Autodesk Inventor part; units mm, degrees
ref_plane "YZ Plane" through (0, 0, 0) normal (1, 0, 0) x (0, 1, 0)
ref_plane "XZ Plane" through (0, 0, 0) normal (0, 1, 0) x (-1, 0, 0)
ref_plane "XY Plane" through (0, 0, 0) normal (0, 0, 1) x (1, 0, 0)
sketch "Szkic1" plane through (0, 0, 0) normal (0, 0, 1) x (1, 0, 0)
  circle A0 centre (0, 0) radius 10
  dimension "d0" = 20
extrude "Wyciągnięcie proste1" add sketch "Szkic1" along normal blind 430
shell "Skorupa1" thickness 2 removed faces 2 at (-1.182, 3.1167, 430) at (-1.182, 3.1167, 0)
sketch "Szkic2" plane through (0, 0, 0) normal (1, 0, 0) x (0, 1, 0)
  line L0 (-34.5081, 100) -> (42.8278, 100)
  line L1 (-10, 0) -> (10, 0)
  line L2 (10, 430) -> (-10, 430)
  point P0 (0, 0)
  dimension "d4" = 100
bend part "Gięcie części1" radius 25.4648 angle 45 line through (0, -34.5081, 100) along (0, 1, 0) centre toward (1, 0, 0) moving side (0, 0, -1) both sides no
sketch "Szkic3" plane through (0, 0, 0) normal (1, 0, 0) x (0, 1, 0)
  line L0 (-35.2697, 330) -> (39.6293, 330)
  line L1 (10, 430) -> (-10, 430)
  point P0 (0, 0)
  dimension "d8" = 100
bend part "Gięcie części2" radius 25.4648 angle 45 line through (0, -35.2697, 330) along (0, 1, 0) centre toward (1, 0, 0) moving side (0, 0, 1) both sides no
sketch "Szkic4" plane through (0, 0, 0) normal (0, 1, 0) x (-1, 0, 0)
  line L0 (-71.0981, 32.4962) -> (-56.9559, 18.3541) construction
  line L1 (-56.9559, 18.3541) -> (-0.3874, 74.9226) construction
  line L2 (-56.9559, 18.3541) -> (-56.9559, 46.6383)
  line L3 (-71.0981, 32.4962) -> (-14.5295, 89.0647) construction
  line L4 (-56.9559, 46.6383) -> (-71.0981, 32.4962)
  line L5 (-71.0981, 32.4962) -> (-56.9559, 18.3541)
  line L6 (-56.9559, 411.6459) -> (-71.0981, 397.5038) construction
  line L7 (-14.5295, 340.9353) -> (-71.0981, 397.5038) construction
  line L8 (-0.3874, 355.0774) -> (-56.9559, 411.6459) construction
  line L9 (-56.9559, 411.6459) -> (-56.9559, 383.3617)
  line L10 (-56.9559, 383.3617) -> (-71.0981, 397.5038)
  line L11 (-71.0981, 397.5038) -> (-56.9559, 411.6459)
  point P0 (0, 0)
extrude "Wyciągnięcie proste3" cut sketch "Szkic4" along normal mid plane 32
equation "\"PromieńGięcia\" = Grubość"
equation "\"SzerokośćGięciaPodcięcia\" = Grubość"
equation "\"GłębokośćGięciaPodcięcia\" = 0.5 * Grubość"
equation "\"RozmiarPodcięciaNarożnika\" = 4 * Grubość"
equation "\"MinimalnaPozostałość\" = 2 * Grubość"
equation "\"PromieńPrzejścia\" = PromieńGięcia"
equation "\"Rozmiar_promienia_Jacobiego\" = Grubość"
equation "\"Wielk_odstępu\" = Grubość"
properties part number "Rura_poprzeczna_wygieta" material "Aluminium AW-7020"
Can you work these out from the model? Positions are in its coordinate system, mm. A direction names the side the tool comes from. Give positions to 0.01 mm unless a question says otherwise; leave off trailing zeros. Order: outer loops, then holes, each group sorted by start corner. A loop starts at its lowest first (then second) coordinate and runs counter-clockwise, first axis right, second up. Notation, with made-up numbers: M 25,86 L 36,86 A16 ccw 36,109 Z; hole C 88.5,-13 d4. An arc over 180 degrees is marked long. One line per question, with ' | ' between items.
Item 1: We'd pull the mould along X, two halves only. Please class faces 3 (the face through (-1.73, 7.81, 213.39)), 4 (the face through (56.956, -8.2, 32.4)), 5 (the face through (29.81, -0.35, 48.34)), 6 (the face through (22.789, -0.44, 52.534)): released by +X, released by -X, zero draft, split by the parting line, or undercut.
Answer block:
face 3: undercut | face 4: released by +X | face 5: undercut | face 6: split by the parting line
Item 2: Suppose I cut it at B-B, the plane y = 4.75. Write out the boundary of the cut face in (x, z).
Answer block:
outline: M -8.8,100 A34.26 ccw 1.24,75.77 L 56.96,20.05 L 56.96,23.39 L 2.91,77.44 A31.9 cw -6.44,100 L -6.44,330 A31.9 cw 2.91,352.56 L 56.96,406.61 L 56.96,409.95 L 1.24,354.23 A34.26 ccw -8.8,330 Z; M 6.44,100 A19.03 ccw 12.01,86.55 L 56.96,41.6 L 56.96,44.94 L 13.68,88.22 A16.66 cw 8.8,100 L 8.8,330 A16.66 cw 13.68,341.78 L 56.96,385.06 L 56.96,388.4 L 12.01,343.45 A19.03 ccw 6.44,330 Z
Item 3: Suppose I cut it at A-A, the plane z = 207. Write out the boundary of the cut face in (x, y).
Answer block:
outline: C 0,0 d20; hole C 0,0 d16
Item 4: Suppose I cut it at C-C, the plane x = 39.5. Give the number of separate pieces and of enclosed holes in the cut face, then the cut area to 3 significant figures.
Answer block:
separate pieces: 2 | enclosed holes: 2 | area: 320 mm2
Item 5: Please list where these lines run through material, in increasing order: L1, parallel to X at y = 0, z = 167; L2, parallel to Z at x = 38.5, y = 5; L3, parallel to Z at x = 36, y = 3.5.
Answer block:
L1: x = -10 to -8, 8 to 10 | L2: z = 38.7 to 42.12, 59.78 to 63.2, 366.8 to 370.22, 387.88 to 391.3 | L3: z = 40.2 to 43.28, 63.63 to 66.7, 363.3 to 366.37, 386.72 to 389.8
Item 6: For faces 1 (the face through (56.956, -8.2, 397.6)), 2 (the face through (-2.17, 9.76, 213.39)), which set-ups out of +Z, -Z, +X, -X, +Y, -Y let a thin tool reach every point of the face, with its end or its side?
Answer block:
face 1: +Z, -Z, +X, +Y, -Y | face 2: none
Item 7: I'm going to push flat-ended pins straight in: pin 1 Ø1 at (x, y) = (25.5, -6.5) entering from -Z; pin 2 Ø4 at (x, y) = (31.5, -1.5) entering from +Z; pin 3 Ø3 at (x, y) = (49.5, 6) entering from -Z. Where does each tip first touch, or does it pass through?
Answer block:
pin 1: stops at z = 52.44 | pin 2: stops at z = 388.07 | pin 3: stops at z = 26.58
